The listing builds one solid part. Answer for the finished solid, in the listing's coordinates (mm). A direction names the side the tool comes from. Coordinates: 2 decimals unless noted, no trailing zeros. Order: outer loops, then holes, each group sorted by start corner. A loop starts at its lowest first (then second) coordinate and runs counter-clockwise, first axis right, second up. Notation, with made-up numbers: (-25.75, 87.25) -> (28.25, 87.25) arc R22 ccw to (28.25, 111.25) -> close; hole circle Ø6 at (0.5, 2.5). An arc over 180 degrees is marked (long way). Write each question's results on one line, items separated by ' | '. Start each with the question number.
(1) Given pin 1 (12 mm diameter, centred on x = 35, y = 191, fed in from -Z); pin 2 (8 mm diameter, centred on x = 100, y = 294, fed in from +Z); pin 3 (4 mm diameter, centred on x = 195, y = 40, fed in from +Z), each flat-ended and moving along its own axis, determine where each tip first touches the part or whether it passes through.
(2) A tool of negligible diameter and unlimited length cuts with its end or side. For faces 1 (the face through (10.496, 40.209, 7.465)), 2 (the face through (196.341, 101.767, 2.465)), from which of +Z, -Z, +X, -X, +Y, -Y can it reach the whole face along a straight path? Write none if from no direction.
(3) The part is cut by section A-A, the plane x = 5. Give the vertices of the cut face in (y, z).
(4) Determine the mould class of faces 3 (the face through (145.72, 245.84, 7.46)), 4 (the face through (0, 177, 5)), 5 (the face through (99, 0, 5)), 6 (the face through (4.846, 43.497, 2.465)) for opening direction Y: +Y half, -Y half, draft (parallel to the pull), parting line (faces both ways), or undercut.
(5) Straight lines are drawn through the part: L1, parallel to X at y = 250, z = 1.75; L2, parallel to Y at x = 5, z = 7.6; L3, parallel to X at y = 8.75, z = 5. For each, find the intervals that lie inside material, in ascending order.
Autodesk Inventor part; units mm, degrees
ref_plane "YZ Plane" through (0, 0, 0) normal (1, 0, 0) x (0, 1, 0)
ref_plane "XZ Plane" through (0, 0, 0) normal (0, 1, 0) x (-1, 0, 0)
ref_plane "XY Plane" through (0, 0, 0) normal (0, 0, 1) x (1, 0, 0)
sketch "Sketch1" plane through (0, 0, 0) normal (0, 0, 1) x (1, 0, 0)
  line L0 (0, 0) -> (200, 0)
  line L1 (200, 0) -> (200, 350)
  line L2 (200, 350) -> (0, 350)
  line L3 (0, 350) -> (0, 0)
  dimension "d0" = 200
  dimension "d1" = 350
extrude "Extrusion1" add sketch "Sketch1" along normal blind 10
sketch "Sketch2" plane through (0, 0, 10) normal (0, 0, 1) x (1, 0, 0)
  circle A0 centre (144, 250) radius 2.067
  circle A1 centre (176, 250) radius 2.067
  circle A2 centre (100, 326) radius 2.067
  circle A3 centre (100, 294) radius 2.067
  circle A4 centre (56, 250) radius 2.067
  circle A5 centre (24, 250) radius 2.067
  circle A6 centre (100, 206) radius 2.067
  circle A7 centre (100, 174) radius 2.067
  point P0 (0, 0)
hole "Hole1" at (24, 250, 10) at (56, 250, 10) at (100, 294, 10) at (100, 326, 10) at (144, 250, 10) at (176, 250, 10) at (100, 206, 10) at (100, 174, 10) direction (0, 0, -1) diameter 6 end through all counterbore diameter 9 counterbore depth 5
sketch "Sketch3" plane through (0, 0, 0) normal (0, -1, 0) x (1, 0, 0)
  line L0 (0, 0) -> (0, 10)
  line L1 (0, 5) -> (200, 5)
  line L2 (200, 0) -> (200, 10)
  circle A0 centre (24, 5) radius 3
  circle A1 centre (56, 5) radius 3
  circle A2 centre (144, 5) radius 3
  circle A3 centre (176, 5) radius 3
  dimension "d11" = 6
  dimension "d12" = 6
  dimension "d13" = 6
  dimension "d14" = 6
  dimension "d15" = 24
  dimension "d16" = 56
  dimension "d17" = 24
  dimension "d18" = 56
hole "Hole2" at (24, 0, 5) at (56, 0, 5) at (144, 0, 5) at (176, 0, 5) direction (0, 1, 0) diameter 4.917 depth 17.1
sketch "Sketch4" plane through (0, 0, 10) normal (0, 0, 1) x (1, 0, 0)
  circle A0 centre (195, 40) radius 2.5941
  circle A1 centre (195, 105) radius 2.5941
  circle A2 centre (5, 105) radius 2.5941
  circle A3 centre (5, 40) radius 2.5941
  point P0 (0, 0)
hole "Hole3" at (5, 105, 10) at (5, 40, 10) at (195, 105, 10) at (195, 40, 10) direction (0, 0, -1) diameter 7 end through all counterbore diameter 11 counterbore depth 5
properties part number "290x200(10li)"
Established:
1) pin 1: stops at z = 0 | pin 2: stops at z = 5 | pin 3: passes through
2) face 1: +Z | face 2: +Z, -Z
3) outline: (0, 0) -> (36.5, 0) -> (36.5, 5) -> (34.5, 5) -> (34.5, 10) -> (0, 10) -> close; (43.5, 0) -> (101.5, 0) -> (101.5, 5) -> (99.5, 5) -> (99.5, 10) -> (45.5, 10) -> (45.5, 5) -> (43.5, 5) -> close; (108.5, 0) -> (350, 0) -> (350, 10) -> (110.5, 10) -> (110.5, 5) -> (108.5, 5) -> close
4) face 3: undercut | face 4: draft | face 5: -Y half | face 6: undercut
5) L1: x = 0 to 21, 27 to 53, 59 to 141, 147 to 173, 179 to 200 | L2: y = 0 to 34.5, 45.5 to 99.5, 110.5 to 350 | L3: x = 0 to 21.54, 26.46 to 53.54, 58.46 to 141.54, 146.46 to 173.54, 178.46 to 200
